The model under review builds one solid part; all positions refer to its coordinate system, in mm. Coordinates: 2 decimals unless noted, no trailing zeros. Order: outer loops, then holes, each group sorted by start corner. A loop starts at its lowest first (then second) coordinate and runs counter-clockwise, first axis right, second up. Notation, with made-up numbers: (43, 19.5) -> (74, 19.5) arc R24 ccw to (74, 30.5) -> close; hole circle Ø5 at (52.5, 18.25). An arc over 180 degrees is marked (long way). Use CSV: the item, a comma, the result in double quotes. Start each with the question number.
Solid Edge part; units mm, degrees
sketch "Sketch1" plane through (0, 0, 0) normal (1, 0, 0) x (0, 1, 0)
  circle A0 centre (-15, 0) radius 3
  circle A1 centre (15, 0) radius 3
  line L0 (20, -5) -> (-20, -5)
  line L1 (-20, -5) -> (-20, 5)
  line L2 (-20, 5) -> (20, 5)
  line L3 (20, 5) -> (20, -5)
  dimension "D1" = 20
  dimension "D2" = 20
extrude "Protrusion1" add sketch "Sketch1" along normal blind 50
sketch "Sketch2" plane through (25, 0, 5) normal (0, 0, 1) x (1, 0, 0)
  circle A0 centre (-15, 0) radius 2.5
  circle A1 centre (17.5, 0) radius 2.5
extrude "Cutout1" cut sketch "Sketch2" against normal up to next
sketch "Sketch3" plane through (50, 0, 0) normal (1, 0, 0) x (0, 1, 0)
  line L0 (-20, -5) -> (20, -5)
  line L1 (20, -5) -> (20, 5)
  line L2 (20, 5) -> (-20, 5)
  line L3 (-20, 5) -> (-20, -5)
  circle A0 centre (15, 0) radius 3
  circle A1 centre (-15, 0) radius 3
extrude "ExtrudedProtrusion_4" add sketch "Sketch3" along normal blind 5
properties material "ABS Plastic, high impact"
Q1. Draft analysis for pull direction Y (two halves, no side actions). For faces 1 (the flat face through (27, 20, 0)), 2 (the flat face through (0, 0, 0)), 3 (the cylindrical face through (7.5, 0.1, 0.1)), state which applies: +Y half, -Y half, draft (parallel to the pull), parting line (faces both ways), or undercut.
Q2. Add section A-A, the plane x = 10. State the section outline as (y, z) points, then the cut area to 3 significant figures.
Q3. Clearance check with a flat-ended pin moving along its axis: pin 1 Ø6.5 at (x, y) = (10, 0) entering from +Z. State where the tip first meets the part, or that it passes through.
Q4. To check wall thickness, follow probe 1 along Y at (x, z) = (47.5, -0.25); probe 2 along Y at (x, z) = (42.5, -1.25); probe 3 along Z at (x, y) = (45.5, 15). State the ranges of each line that lie inside material, in increasing order.
Q5. Add section B-B, the plane y = 15. State the section outline as (x, z) points, then the cut area to 3 significant figures.
Q6. Add section D-D, the plane y = 0. State the section outline as (x, z) points.
Q7. Add section C-C, the plane z = 0. State the section outline as (x, y) points, then the cut area to 3 significant figures.
Answer block:
1,face 1,"+Y half"
1,face 2,"draft"
1,face 3,"undercut"
2,outline,"(-20, -5) -> (-2.5, -5) -> (-2.5, 5) -> (-20, 5) -> close; (2.5, -5) -> (20, -5) -> (20, 5) -> (2.5, 5) -> close; hole circle Ø6 at (-15, 0); hole circle Ø6 at (15, 0)"
2,area,"293 mm²"
3,pin 1,"stops at z = 5"
4,probe 1,"y = -20 to -17.99, -12.01 to 12.01, 17.99 to 20"
4,probe 2,"y = -20 to -17.73, -12.27 to -2.5, 2.5 to 12.27, 17.73 to 20"
4,probe 3,"z = -5 to -3, 3 to 5"
5,outline,"(0, -5) -> (55, -5) -> (55, -3) -> (0, -3) -> close; (0, 3) -> (55, 3) -> (55, 5) -> (0, 5) -> close"
5,area,"220 mm²"
6,outline,"(0, -5) -> (7.5, -5) -> (7.5, 5) -> (0, 5) -> close; (12.5, -5) -> (40, -5) -> (40, 5) -> (12.5, 5) -> close; (45, -5) -> (55, -5) -> (55, 5) -> (45, 5) -> close"
7,outline,"(0, -20) -> (55, -20) -> (55, -18) -> (0, -18) -> close; (0, -12) -> (55, -12) -> (55, 12) -> (0, 12) -> close; (0, 18) -> (55, 18) -> (55, 20) -> (0, 20) -> close; hole circle Ø5 at (10, 0); hole circle Ø5 at (42.5, 0)"
7,area,"1,500 mm²"
